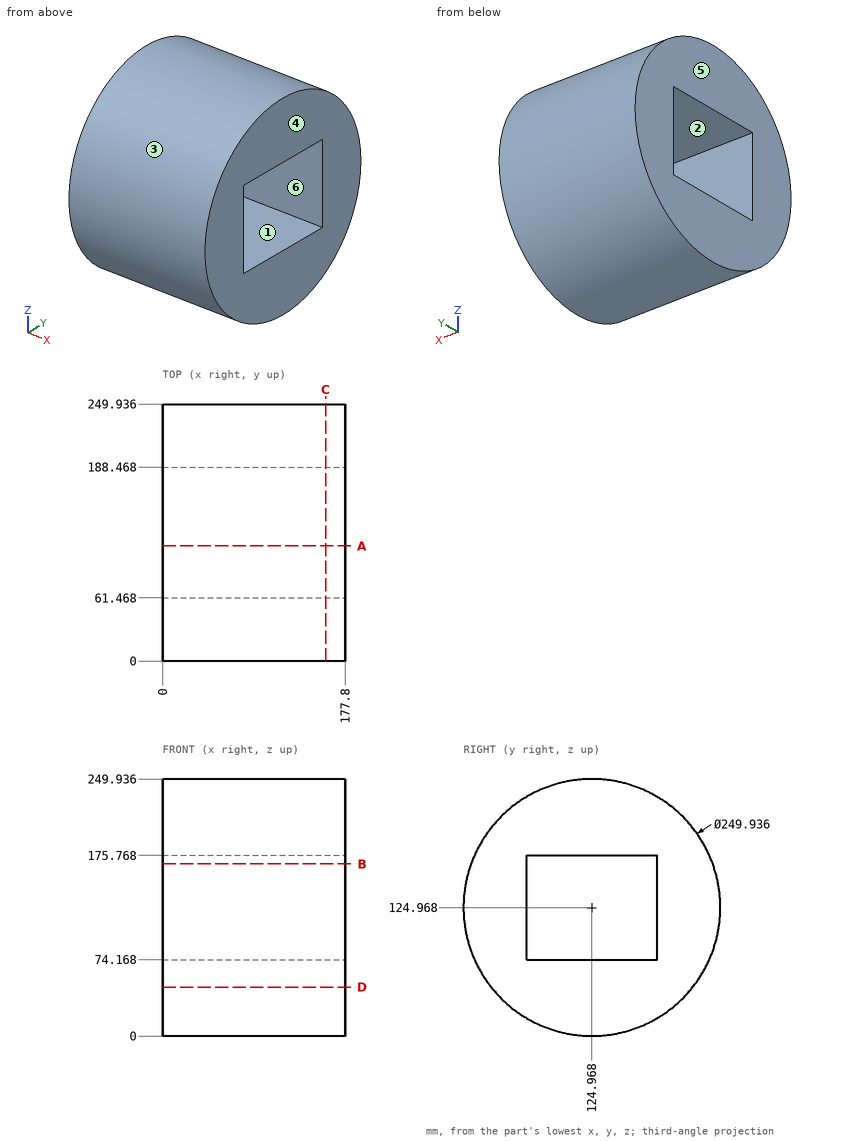
Part print with two shaded views. Sizes in mm from the minimum x, y, z corner. A direction names the side the tool comes from. Give positions to 0.01 mm unless a question says otherwise; leave off trailing zeros. Order: outer loops, then holes, each group sorted by start corner. A loop starts at its lowest first (then second) coordinate and runs counter-clockwise, first axis right, second up. Notation, with made-up numbers: M -29,85 L -3,85 A22 cw -3,112 Z; hole C -24,10.5 d1. An arc over 180 degrees is marked long. Write item = value, one per line.
Q1. Cut at D-D, the plane z = 47.5. List the corners of the cut face in (x, y).
Derived:
outline = M 0,26.91 L 177.8,26.91 L 177.8,223.03 L 0,223.03 Z
Q2. Cut at B-B, the plane z = 167.5. List the corners of the cut face in (x, y).
Derived:
outline = M 0,7.46 L 177.8,7.46 L 177.8,61.47 L 0,61.47 Z; M 0,188.47 L 177.8,188.47 L 177.8,242.48 L 0,242.48 Z
Q3. Drill centre lines: line 1 (Y direction, x = 115, z = 101); line 2 (Z direction, x = 120.5, y = 165); line 3 (Z direction, x = 150, y = 94). Where is each one in solid material? Low to high. Write a range as [from, to].
Derived:
line_1 = [2.32, 61.47], [188.47, 247.62]
line_2 = [6.59, 74.17], [175.77, 243.35]
line_3 = [3.9, 74.17], [175.77, 246.04]
Q4. Flat gauge pins, fed straight in: pin 1 (2 mm diameter, centred on x = 99, z = 172, fed in from -Y); pin 2 (3 mm diameter, centred on x = 152.5, y = 64.5, fed in from +Z); pin 3 (1 mm diameter, centred on x = 49.5, y = 131, fed in from -Z). Where does each tip first touch, or does it go through?
Derived:
pin_1 = 8.79
pin_2 = 235.15
pin_3 = 0.12
Q5. Two-plate mould, pull along Y, no slides. Class the marked faces 1, 2, 3 and 4: pulls with the +Y half, pulls with the -Y half, needs draft (parallel to the pull), parting line crosses it, or undercut.
Derived:
face_1 = undercut
face_2 = undercut
face_3 = parting line crosses it
face_4 = needs draft
Q6. Cut at C-C, the plane x = 158.5. List the corners of the cut face in (y, z).
Derived:
outline = C 124.97,124.97 d249.94; hole M 61.47,74.17 L 188.47,74.17 L 188.47,175.77 L 61.47,175.77 Z
Q7. Cut at A-A, the plane y = 112. List the corners of the cut face in (x, z), then the cut area to 3 significant figures.
Derived:
outline = M 0,0.67 L 177.8,0.67 L 177.8,74.17 L 0,74.17 Z; M 0,175.77 L 177.8,175.77 L 177.8,249.26 L 0,249.26 Z
area = 26,100 mm2
Q8. Tool access for the marked faces 5 and 6: list every direction of +Z, -Z, +X, -X, +Y, -Y with a clear straight run to the whole face (end or side of a thin tool).
Derived:
face_5 = +Z, -Z, -X, +Y, -Y
face_6 = +X, -X
